```python
from build123d import *

# Parameters (mm, degrees)
FILLET1_R               = 3
CUT_EXTRUDE1_REACH      = 62
CUT_EXTRUDE1_END_RADIUS = 16
SKETCH4_R               = 1.5
SKETCH5_R               = 3.75
CUT_EXTRUDE2_DEPTH      = 62.846584425
CIRPATTERN1_COUNT       = 8
FILLET3_R               = 2.5


with BuildPart() as part:
    # Sketch2 → Base-Revolve (revolve)
    with BuildSketch(Plane.XY, mode=Mode.PRIVATE) as base_revolve_sk:
        Polygon((20, 40), (-20, 40), (-20, 37), (-5, 35), (-5, 16), (-20, 16), (-20, 8), (20, 8), (20, 16), (5, 16), (5, 35), (20, 37), align=None)
    revolve(base_revolve_sk.sketch.rotate(Axis((-102.775053376, 0, 0), (1, 0, 0)), 90), axis=Axis((-102.775053376, 0, 0), (1, 0, 0)))

    # Fillet1
    fillet1_edges = [part.edges().sort_by_distance(p)[0] for p in [
        (5, 0, -35),
        (-5, 0, -35),
    ]]
    fillet(fillet1_edges, radius=FILLET1_R)

    # Cut-Extrude1: up to this cylinder (the profile starts inside it)
    cut_extrude1_end = Plane(origin=(14, 0, 0), z_dir=(-1, 0, 0)) * Cylinder(CUT_EXTRUDE1_END_RADIUS, 157, mode=Mode.PRIVATE)
    # Sketch4 → Cut-Extrude1 (cut, up to the surface)
    with BuildSketch(Plane(origin=(0, 0, 0), x_dir=(1, 0, 0), z_dir=(0, 1, 0)), mode=Mode.PRIVATE) as cut_extrude1_sk1:
        with Locations(Location((14, 0, 0), (0, 0, 90))):
            Circle(SKETCH4_R)
    cut_extrude1_tool1 = extrude(cut_extrude1_sk1.sketch, amount=CUT_EXTRUDE1_REACH, mode=Mode.PRIVATE) & cut_extrude1_end
    cut_extrude1 = cut_extrude1_tool1.solids().sort_by_distance((14, 0, 0))[0]
    add(cut_extrude1, mode=Mode.SUBTRACT)

    # Mirror1: Cut-Extrude1 across plane
    add(cut_extrude1.mirror(Plane(origin=(0, 0, 0), x_dir=(0, 0, 1), z_dir=(1, 0, 0))), mode=Mode.SUBTRACT)

    # Sketch5 → Cut-Extrude2 (cut, through all)
    with BuildSketch(Plane(origin=(5, 0, 0), x_dir=(0, 0, -1), z_dir=(1, 0, 0))):
        with Locations((-17.67766953, 17.67766953)):
            Circle(SKETCH5_R)
    cut_extrude2 = extrude(amount=-CUT_EXTRUDE2_DEPTH, mode=Mode.SUBTRACT)

    # CirPattern1: Cut-Extrude2 ×8 about axis
    cirpattern1_axis = Axis((0, 0, 0), (1, 0, 0))
    for i in range(1, CIRPATTERN1_COUNT):
        add(cut_extrude2.rotate(cirpattern1_axis, i * 360 / CIRPATTERN1_COUNT), mode=Mode.SUBTRACT)

    # Fillet3
    fillet3_edges = [part.edges().sort_by_distance(p)[0] for p in [
        (20, 0, -16),
        (-20, 0, -16),
    ]]
    fillet(fillet3_edges, radius=FILLET3_R)


solid = part.part
```
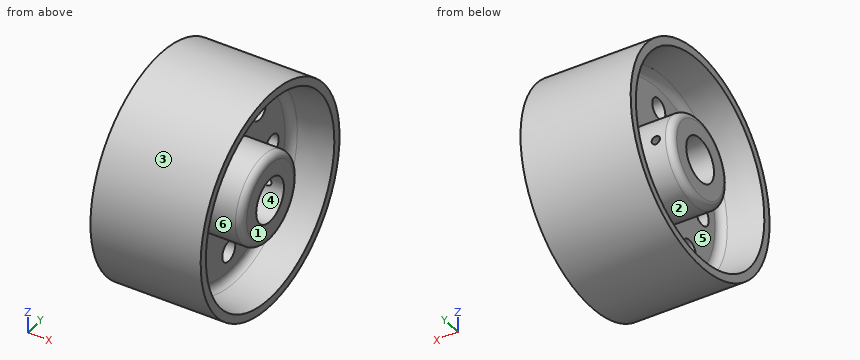
Geometry: final body of the model. Coordinates: model frame, mm. Face numbers are marked on the shaded views. A direction names the side the tool comes from. Coordinates: 2 decimals unless noted, no trailing zeros. Loops run counter-clockwise (first coordinate to the right, second up) from the corner with the lowest first, then second, coordinate; pieces in that order, holes last. Notation, with made-up numbers: (-8, 35) -> (42, 35) arc R29 ccw to (42, 58) -> close; hole circle Ø8 at (87.5, 48.5). An arc over 180 degrees is marked (long way). Use a Markdown table: item, result. Add a question column.
(1) Mould query, pull axis Z, two halves, no side actions, for the marked faces 1, 2 and 3. Classes: pulls with the +Z half, pulls with the -Z half, needs draft (parallel to the pull), parting line crosses it, or undercut.
(2) Line query: line 1 along Y through (x, z) = (-2.25, 0); line 2 along X through (y, z) = (12, 0); line 3 along Z through (x, y) = (17, -14). Output: solid intervals per line, ascending.
(3) Section query B-B, the plane x = 14. Return loops of the section in (y, z), plus the area to 3 significant figures.
(4) Pin query (flat end, axial travel): pin 1 Ø1 at (x, y) = (9, 1.5) entering from +Z; pin 2 Ø3 at (x, y) = (7.5, -24.5) entering from +Z; pin 3 Ø1 at (x, z) = (9.5, 4.5) entering from -Y. Return the tip coordinate at first contact, or that it passes through.
(5) Access query for the marked faces 4, 5 and 6. Directions: +Z, -Z, +X, -X, +Y, -Y. A direction counts if a zero-diameter tool reaches every point of the face in a straight line with its end or side. Return the directions, or none.
(6) Section query A-A, the plane y = 0. State how many separate pieces and enclosed holes the cut face has, plus the area to 3 significant figures.
Answer:
| question | item | result |
|---|---|---|
| 1 | face 1 | needs draft |
| 1 | face 2 | undercut |
| 1 | face 3 | parting line crosses it |
| 2 | line 1 | y = -40 to -28.75, -21.25 to -8, 8 to 21.25, 28.75 to 40 |
| 2 | line 2 | x = -20 to -15.5, -12.5 to 12.5, 15.5 to 20 |
| 2 | line 3 | z = -37.47 to -33.82, -7.75 to 7.75, 33.82 to 37.47 |
| 3 | outline | circle Ø80 at (0, 0); (7.86, -1.5) arc R8 cw (long way) to (7.86, 1.5) -> (15.93, 1.5) arc R16 ccw (long way) to (15.93, -1.5) -> close; hole circle Ø72.4 at (0, 0) |
| 3 | area | 1,490 mm^2 |
| 4 | pin 1 | stops at z = 39.99 |
| 4 | pin 2 | stops at z = 32.73 |
| 4 | pin 3 | stops at y = -39.8 |
| 5 | face 4 | +X, -X |
| 5 | face 5 | -X |
| 5 | face 6 | +X |
| 6 | separate pieces | 4 |
| 6 | enclosed holes | 0 |
| 6 | area | 1,210 mm^2 |
